CAD build for the part. Positions are in the model's coordinates, mm. Round coordinates to 2 decimals unless told otherwise and drop trailing zeros. Order: outer loops, then holes, each group sorted by start corner. A loop starts at its lowest first (then second) coordinate and runs counter-clockwise, first axis right, second up. Notation, with made-up numbers: M -32,87.5 L -26,87.5 A17 cw -26,107.5 Z; hole C 36,-19 d11. An arc over 180 degrees is marked long. Answer as a JSON object with one key per item and string values.
```python
from build123d import *

# Parameters (mm, degrees)
SKETCH2_W           = 127
SKETCH2_H           = 76.2
BOSS_EXTRUDE1_DEPTH = 6.35
SKETCH3_W           = 25.4
SKETCH3_H           = 6.35
BOSS_EXTRUDE2_DEPTH = 6.35
CUT_EXTRUDE1_DEPTH  = 78.771299333
SKETCH5_R           = 5.588
CUT_EXTRUDE2_DEPTH  = 78.771299333


with BuildPart() as part:
    # Sketch2 → Boss-Extrude1 (new body)
    with BuildSketch(Plane.XY):
        Rectangle(SKETCH2_W, SKETCH2_H)
    extrude(amount=BOSS_EXTRUDE1_DEPTH)

    # Sketch3 → Boss-Extrude2 (add)
    with BuildSketch(Plane.XY.offset(6.35)):
        with Locations((0, 41.275)):
            Rectangle(SKETCH3_W, SKETCH3_H)
        with Locations((50.8, 41.275)):
            Rectangle(SKETCH3_W, SKETCH3_H)
        with Locations((50.8, -41.275)):
            Rectangle(SKETCH3_W, SKETCH3_H)
        with Locations((0, -41.275)):
            Rectangle(SKETCH3_W, SKETCH3_H)
        with Locations((-50.8, -41.275)):
            Rectangle(SKETCH3_W, SKETCH3_H)
        with Locations((-50.8, 41.275)):
            Rectangle(SKETCH3_W, SKETCH3_H)
    extrude(amount=-BOSS_EXTRUDE2_DEPTH)

    # Sketch4 → Cut-Extrude1 (cut, through all)
    with BuildSketch(Plane.XY.offset(6.35)):
        Polygon((-27.432, 38.1), (-23.368, 38.1), (-23.368, 30.48), (-21.971, 30.48), (-21.971, 27.432), (-23.368, 27.432), (-23.368, 22.606), (-27.432, 22.606), (-27.432, 27.432), (-28.829, 27.432), (-28.829, 30.48), (-27.432, 30.48), align=None)
        Polygon((27.432, 38.1), (23.368, 38.1), (23.368, 30.48), (21.971, 30.48), (21.971, 27.432), (23.368, 27.432), (23.368, 22.606), (27.432, 22.606), (27.432, 27.432), (28.829, 27.432), (28.829, 30.48), (27.432, 30.48), align=None)
        Polygon((27.432, -38.1), (23.368, -38.1), (23.368, -30.48), (21.971, -30.48), (21.971, -27.432), (23.368, -27.432), (23.368, -22.606), (27.432, -22.606), (27.432, -27.432), (28.829, -27.432), (28.829, -30.48), (27.432, -30.48), align=None)
        Polygon((-27.432, -38.1), (-23.368, -38.1), (-23.368, -30.48), (-21.971, -30.48), (-21.971, -27.432), (-23.368, -27.432), (-23.368, -22.606), (-27.432, -22.606), (-27.432, -27.432), (-28.829, -27.432), (-28.829, -30.48), (-27.432, -30.48), align=None)
    extrude(amount=-CUT_EXTRUDE1_DEPTH, mode=Mode.SUBTRACT)

    # Sketch5 → Cut-Extrude2 (cut, through all)
    with BuildSketch(Plane.XY.offset(6.35)):
        Circle(SKETCH5_R)
    extrude(amount=-CUT_EXTRUDE2_DEPTH, mode=Mode.SUBTRACT)


solid = part.part
```
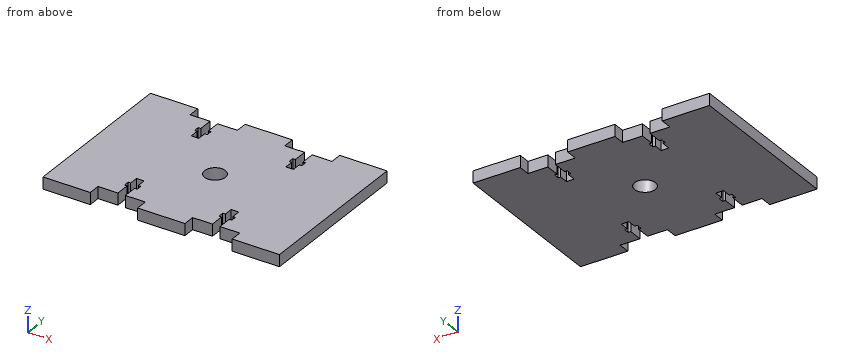
Item 1: Saw through at A-A on y = 0. List the corners of the cut face in (x, z), and give its area (3 significant figures).
Worked answers:
{"outline": "M -63.5,0 L -5.59,0 L -5.59,6.35 L -63.5,6.35 Z; M 5.59,0 L 63.5,0 L 63.5,6.35 L 5.59,6.35 Z", "area": "735 mm2"}
Item 2: Wall check: line 1 along X through (y, z) = (-37.5, 5.5); line 2 along X through (y, z) = (-29.5, 2.75); line 3 along Y through (x, z) = (0, 2.25). Give the ranges that are in metal, low to high. Write a range as [from, to].
Worked answers:
{"line 1": "x = [-63.5, -27.43], [-23.37, 23.37], [27.43, 63.5]", "line 2": "x = [-63.5, -28.83], [-21.97, 21.97], [28.83, 63.5]", "line 3": "y = [-44.45, -5.59], [5.59, 44.45]"}
Item 3: Saw through at C-C on y = 29. List the corners of the cut face in (x, z).
Worked answers:
{"outline": "M -63.5,0 L -28.83,0 L -28.83,6.35 L -63.5,6.35 Z; M -21.97,0 L 21.97,0 L 21.97,6.35 L -21.97,6.35 Z; M 28.83,0 L 63.5,0 L 63.5,6.35 L 28.83,6.35 Z"}
Item 4: Saw through at B-B on x = 0. List the corners of the cut face in (y, z), and give its area (3 significant figures).
Worked answers:
{"outline": "M -44.45,0 L -5.59,0 L -5.59,6.35 L -44.45,6.35 Z; M 5.59,0 L 44.45,0 L 44.45,6.35 L 5.59,6.35 Z", "area": "494 mm2"}
Item 5: Drop flat-ended pins along their axis: pin 1 Ø1.5 at (x, z) = (22.5, 1.5) entering from +Y; pin 2 Ø1 at (x, y) = (-13, 4) entering from -Z; pin 3 Ø0.7 at (x, z) = (28.5, 3) entering from -Y. Give the stop position or say it passes through.
Worked answers:
{"pin 1": "stops at y = 38.1", "pin 2": "stops at z = 0", "pin 3": "stops at y = -38.1"}
